```python
from build123d import *

# Parameters (mm, degrees)
F0_W     = 150.0187367201
F0_H     = 50.0062517822
F1_DEPTH = 15
F4_W     = 134.1393142939
F4_H     = 34.7154848278
F5_DEPTH = 39.6
F6_W     = 8.5336472839
F6_H     = 34.7154848278
F7_DEPTH = 15
F9_D     = 7.5
F11_D    = 7.5


with BuildPart() as f1:
    # F0 (on Top) → F1 (new body)
    with BuildSketch(Plane.XY):
        Rectangle(F0_W, F0_H)
    extrude(amount=F1_DEPTH)

    # F4 (on face) → F5 (cut)
    with BuildSketch(Plane.XY.offset(15)):
        Rectangle(F4_W, F4_H)
    extrude(amount=-F5_DEPTH, mode=Mode.SUBTRACT)

    # F6 (on face) → F7 (join)
    with BuildSketch(Plane.XY.offset(15)):
        Rectangle(F6_W, F6_H)
    extrude(amount=-F7_DEPTH)

    # F9 (through all)
    with Locations(Plane(origin=(0, 25.0031258911, 0), x_dir=(-1, 0, 0), z_dir=(0, 1, 0))):
        with Locations((-58.490190655, 7.2111194022)):
            Hole(F9_D / 2)

    # F11 (through all)
    with Locations(Plane(origin=(0, 25.0031258911, 0), x_dir=(-1, 0, 0), z_dir=(0, 1, 0))):
        with Locations((59.4607852399, 7.0205056109)):
            Hole(F11_D / 2)


solid = f1.part
```
Design review of the part built by this model. Coordinates are the model's own, in mm. A direction names the side the tool comes from. Give positions to 0.01 mm unless a question says otherwise; leave off trailing zeros. Order: outer loops, then holes, each group sorted by start corner. A loop starts at its lowest first (then second) coordinate and runs counter-clockwise, first axis right, second up. Notation, with made-up numbers: (-8, 81.5) -> (0, 81.5) arc R13 cw to (0, 105.5) -> close; hole circle Ø11 at (65, 17). An arc over 180 degrees is marked (long way). Write item = value, one per line. Start each with the question number.
(1) We need section C-C on x = 30.5. Write out the cut boundary in (y, z), plus the area to 3 significant figures.
(2) For faces 1 (the face through (-1, -25.003, 7)), 2 (the face through (67.07, 0, 8)), list the 3-axis set-ups (+Z, -Z, +X, -X, +Y, -Y) from which the entire face can be reached by the end or side of a thin tool; tool diameter is ignored.
(3) To check wall thickness, follow line 1 along X through (y, z) = (11.5, 11.75); line 2 along Y through (x, z) = (8, 5.25); line 3 along Z through (x, y) = (-58.5, -17.5). State the ranges of each line that lie inside material, in increasing order.
(4) We need section B-B on z = 1.5. Write out the cut boundary in (x, y).
(5) We need section A-A on y = -14. Write out the cut boundary in (x, z).
(6) Mouldability with a two-part tool opening along X and no side actions: class faces 3 (the face through (-75.009, 0, 7)), 4 (the face through (-1, 0, 15)), 5 (the face through (-36, 17.358, 8)) as +X half, -X half, draft (parallel to the pull), parting line (faces both ways), or undercut.
(7) We need section D-D on y = -21.5. Write out the cut boundary in (x, z).
(8) For pin 1 (6 mm diameter, centred on x = 58.49, z = 7.21, fed in from +Y), flat-tipped, find the tip position at first contact; note if it passes through.
Numbers:
q1.outline = (-25, 0) -> (-17.36, 0) -> (-17.36, 15) -> (-25, 15) -> close; (17.36, 0) -> (25, 0) -> (25, 15) -> (17.36, 15) -> close
q1.area = 229 mm^2
q2.face_1 = +Z, -Z, +X, -X, -Y
q2.face_2 = +Z, -Z
q3.line_1 = -75.01 to -67.07, -4.27 to 4.27, 67.07 to 75.01
q3.line_2 = -25 to -17.36, 17.36 to 25
q3.line_3 = 0 to 3.4, 10.65 to 15
q4.outline = (-75.01, -25) -> (75.01, -25) -> (75.01, 25) -> (-75.01, 25) -> close; hole (-67.07, -17.36) -> (-4.27, -17.36) -> (-4.27, 17.36) -> (-67.07, 17.36) -> close; hole (4.27, -17.36) -> (67.07, -17.36) -> (67.07, 17.36) -> (4.27, 17.36) -> close
q5.outline = (-75.01, 0) -> (-67.07, 0) -> (-67.07, 15) -> (-75.01, 15) -> close; (-4.27, 0) -> (4.27, 0) -> (4.27, 15) -> (-4.27, 15) -> close; (67.07, 0) -> (75.01, 0) -> (75.01, 15) -> (67.07, 15) -> close
q6.face_3 = -X half
q6.face_4 = draft
q6.face_5 = undercut
q7.outline = (-75.01, 0) -> (75.01, 0) -> (75.01, 15) -> (-75.01, 15) -> close; hole circle Ø7.5 at (-59.46, 7.02); hole circle Ø7.5 at (58.49, 7.21)
q8.pin_1 = through
